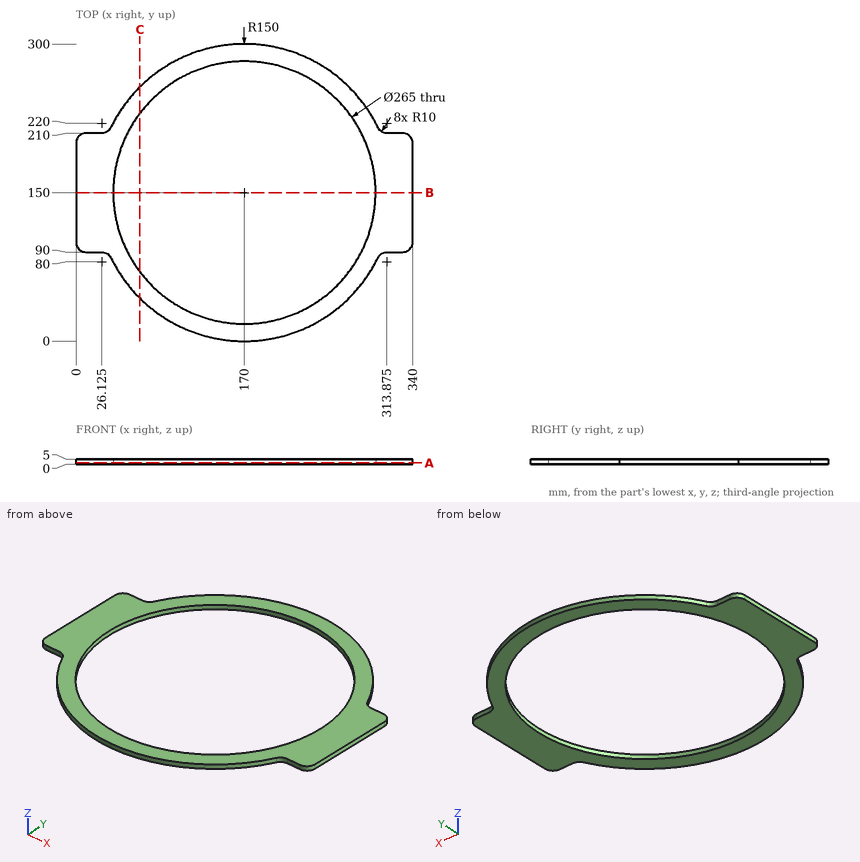
Print and shaded views of the part. All mm, measured from the part's lowest x, y and z. Round coordinates to 2 decimals unless told otherwise and drop trailing zeros. Write each loop counter-clockwise with the first axis right and the second up, starting at its lowest first coordinate (ties: lowest second). Pieces come first, ordered by that corner, then holes. Notation, with made-up numbers: (89.25, 81) -> (144.25, 81) arc R28 ccw to (144.25, 120) -> close; hole circle Ø9 at (-37, 2.5). An arc over 180 degrees is marked (long way). Return JSON: item names as keys, results as strings. Group by question number.
Q1. Probe L1, parallel to X at y = 150, z = 2.35; L2, parallel to Y at x = 186, z = 3.05; L3, parallel to Y at x = 212.5, z = 3.9. List the from-to ranges inside material, lowest first. Write a range as [from, to].
Q2. Saw through at C-C on x = 64.5. Write the cut outline in (y, z).
Q3. Saw through at B-B on y = 150. Write the cut outline in (x, z), plus the area to 3 significant figures.
Q4. Pin check, flat tips, straight feed: pin 1 (2 mm diameter, centred on x = 81, z = 3, fed in from -Y); pin 2 (1 mm diameter, centred on x = 259, z = 3, fed in from -Y); pin 3 (1.5 mm diameter, centred on x = 321.5, z = 3, fed in from -Y). Stop position of each tip, or through.
Q5. Saw through at A-A on z = 1.35. Write the cut outline in (x, y) (3 decimals).
Answer:
{
 "1": {"L1": "[0, 37.5], [302.5, 340]", "L2": "[0.86, 18.47], [281.53, 299.14]", "L3": "[6.15, 24.5], [275.5, 293.85]"},
 "2": {"outline": "(43.37, 0) -> (69.84, 0) -> (69.84, 5) -> (43.37, 5) -> close; (230.16, 0) -> (256.63, 0) -> (256.63, 5) -> (230.16, 5) -> close"},
 "3": {"outline": "(0, 0) -> (37.5, 0) -> (37.5, 5) -> (0, 5) -> close; (302.5, 0) -> (340, 0) -> (340, 5) -> (302.5, 5) -> close", "area": "375 mm2"},
 "4": {"pin 1": "y = 28.53", "pin 2": "y = 28.89", "pin 3": "y = 90"},
 "5": {"outline": "(0, 100) arc R10 ccw to (10, 90) -> (26.125, 90) arc R10 cw to (35.117, 84.375) arc R150 ccw to (304.883, 84.375) arc R10 cw to (313.875, 90) -> (330, 90) arc R10 ccw to (340, 100) -> (340, 200) arc R10 ccw to (330, 210) -> (313.875, 210) arc R10 cw to (304.883, 215.625) arc R150 ccw to (35.117, 215.625) arc R10 cw to (26.125, 210) -> (10, 210) arc R10 ccw to (0, 200) -> close; hole circle Ø265 at (170, 150)"}
}
